The listing builds one solid part. Answer for the finished solid, in the listing's coordinates (mm). A direction names the side the tool comes from. Coordinates: 2 decimals unless noted, no trailing zeros. Order: outer loops, then holes, each group sorted by start corner. A loop starts at its lowest first (then second) coordinate and runs counter-clockwise, first axis right, second up.
Autodesk Inventor part; units mm, degrees
ref_plane "YZ Plane" through (0, 0, 0) normal (1, 0, 0) x (0, 1, 0)
ref_plane "XZ Plane" through (0, 0, 0) normal (0, 1, 0) x (-1, 0, 0)
ref_plane "XY Plane" through (0, 0, 0) normal (0, 0, 1) x (1, 0, 0)
sketch "スケッチ1" plane through (0, 0, 0) normal (0, 1, 0) x (-1, 0, 0)
  circle A0 centre (0, 0) radius 4
  dimension "d0" = 8
extrude "押し出し1" add sketch "スケッチ1" along normal blind 20
sketch "スケッチ2" plane through (0, 20, 0) normal (0, 1, 0) x (1, 0, 0)
  point P0 (0, 0)
  point P1 (0, 0)
hole "穴1" at (0, 20, 0) direction (0, -1, 0) diameter 3.242 depth 6 tip angle 118
sketch "スケッチ3" plane through (0, 0, 0) normal (0, -1, 0) x (1, 0, 0)
  circle A0 centre (0, 0) radius 1.621
hole "穴2" at (0, 0, 0) direction (0, 1, 0) diameter 3.242 depth 6 tip angle 118
properties part number "base_part3" material "アルミニウム 6061"
1) Section B-B (x = -3.25) is taken. Give the vertices of the cut face in (y, z).
2) Section A-A (y = 5) is taken. Give the vertices of the cut face in (x, z), then the cut area to 3 significant figures.
3) Each of these flat-tipped pins is pushed along its axis until it touches: P1, Ø1, axis at x = 1, y = 17.5, coming from the +Z side; P2, Ø1.5, axis at y = 16.5, z = 2.5, coming from the +X side; P3, Ø2, axis at x = 2, y = 4, coming from the +Z side. Where does it stop, or does it pass through?
4) Consider L1, parallel to Z at x = 0, y = 17.75; L2, parallel to Z at x = -1.25, y = 5.75; L3, parallel to X at y = 16.25, z = -3.25. Determine where each line is inside the solid, lowest interval first.
5) A tool of negligible diameter and unlimited length cuts with its end or side. For faces 4 (the face through (1.438, 16.958, 0.748)), 5 (the face through (-0.275, 6.805, 0.061)), from which of +Z, -Z, +X, -X, +Y, -Y can it reach the whole face along a straight path? Write none if from no direction.
6) Determine the mould class of faces 1 (the face through (0.867, 9.86, 3.905)), 2 (the face through (1.438, 3.042, -0.748)), 3 (the face through (-2, 0, 0)) for opening direction Z: released by +Z, released by -Z, zero draft, split by the parting line, or undercut.
Filled sheet:
1. outline: (0, -2.33) - (20, -2.33) - (20, 2.33) - (0, 2.33) - close
2. outline: circle Ø8 at (0, 0); hole circle Ø3.24 at (0, 0)
2. area: 42.0 mm2
3. P1: stops at z = 3.97
3. P2: stops at x = 3.6
3. P3: stops at z = 3.87
4. L1: z = -4 to -1.62, 1.62 to 4
4. L2: z = -3.8 to -1.03, 1.03 to 3.8
4. L3: x = -2.33 to 2.33
5. face 4: +Y
5. face 5: -Y
6. face 1: split by the parting line
6. face 2: undercut
6. face 3: zero draft
